from build123d import *

# Parameters (mm, degrees)
F1_DEPTH = 317.5


with BuildPart() as f1:
    # F0 (on Front) → F1 (new body, symmetric)
    with BuildSketch(Plane.XZ):
        with BuildLine():
            Line((53.8411306598, 32.0202162549), (31.6161306598, 32.0202162549))
            Line((31.6161306598, 32.0202162549), (41.3843568915, -37.8297837451))
            ThreePointArc((41.3843568915, -37.8297837451), (47.6127437756, -45.416592874), (53.8411306598, -37.8297837451))
            Line((53.8411306598, -37.8297837451), (53.8411306598, 32.0202162549))
        make_face()
        Polygon((3.0411306598, 38.3702162549), (3.0411306598, 32.0202162549), (31.6161306598, 32.0202162549), (53.8411306598, 32.0202162549), (53.8411306598, 38.3702162549), align=None)
        Polygon((-47.7588693402, 38.3702162549), (-47.7588693402, 32.0202162549), (-25.5338693402, 32.0202162549), (3.0411306598, 32.0202162549), (3.0411306598, 38.3702162549), align=None)
        with BuildLine():
            Line((-25.5338693402, 32.0202162549), (-47.7588693402, 32.0202162549))
            Line((-47.7588693402, 32.0202162549), (-47.7588693402, -37.8297837451))
            ThreePointArc((-47.7588693402, -37.8297837451), (-41.4088693402, -44.1797837451), (-35.0588693402, -37.8297837451))
            Line((-35.0588693402, -37.8297837451), (-25.5338693402, 32.0202162549))
        make_face()
    extrude(amount=F1_DEPTH, both=True)


solid = f1.part
Build history of the part. All positions in model axes, mm. A direction names the side the tool comes from. Round coordinates to 2 decimals unless told otherwise and drop trailing zeros. Write each loop counter-clockwise with the first axis right and the second up, starting at its lowest first coordinate (ties: lowest second). Pieces come first, ordered by that corner, then holes. Notation, with made-up numbers: (38, -33.5) - (45, -33.5) arc R30 cw to (45, -10.5) - close; hole circle Ø11 at (84, 77). An arc over 180 degrees is marked (long way). One line per question, with ' | ' between items.
1. Mould opens along X. For faces 3 (the face through (47.456, -4.445, -45.415)), 4 (the face through (4, -4, 38.37)), 5 (the face through (53.841, -4, 0)) say: released by +X, released by -X, zero draft, split by the parting line, or undercut.
Results are:
face 3: undercut | face 4: zero draft | face 5: released by +X
2. Drop flat-ended pins along their axis: pin 1 Ø5 at (x, y) = (16.5, 50) entering from -Z; pin 2 Ø1.5 at (y, z) = (32.5, -24.5) entering from +X. Give the stop position or say it passes through.
Results are:
pin 1: z = 32.02 | pin 2: x = 53.84
3. Band-saw the part on B-B, the plane y = 35. Write the cut outline in (x, z).
Results are:
outline: (-47.76, -37.83) arc R6.35 ccw to (-35.06, -37.83) - (-25.53, 32.02) - (31.62, 32.02) - (41.38, -37.83) arc R6.35 ccw (long way) to (53.84, -37.83) - (53.84, 38.37) - (-47.76, 38.37) - close
4. Band-saw the part on A-A, the plane z = -28. Write the cut outline in (x, y).
Results are:
outline: (-47.76, -317.5) - (-33.72, -317.5) - (-33.72, 317.5) - (-47.76, 317.5) - close; (40.01, -317.5) - (53.84, -317.5) - (53.84, 317.5) - (40.01, 317.5) - close
5. Tool access for faces 1 (the face through (2, 317.5, 34)), 2 (the face through (36.432, -4.445, -2.416)): list every direction of +Z, -Z, +X, -X, +Y, -Y with a clear straight run to the whole face (end or side of a thin tool).
Results are:
face 1: +Z, -Z, +X, -X, +Y | face 2: -Z, +Y, -Y
6. Drill centre lines: line 1 along X through (y, z) = (-269, -37); line 2 along Z through (x, y) = (-14, 185); line 3 along X through (y, z) = (281, 14.5). Where is each one in solid material? Low to high. Write a range as from..to.
Results are:
line 1: -47.76..-34.95, 41.27..53.84 | line 2: 32.02..38.37 | line 3: -47.76..-27.92, 34.07..53.84
7. Band-saw the part on C-C, the plane z = 2. Write the cut outline in (x, y).
Results are:
outline: (-47.76, -317.5) - (-29.63, -317.5) - (-29.63, 317.5) - (-47.76, 317.5) - close; (35.81, -317.5) - (53.84, -317.5) - (53.84, 317.5) - (35.81, 317.5) - close
